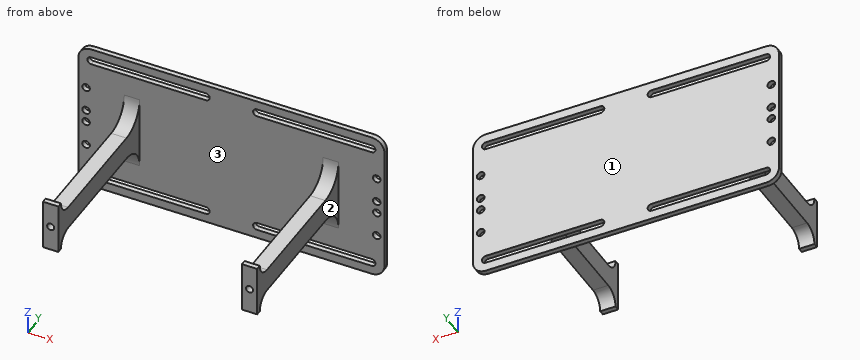
```python
from build123d import *

# Parameters (mm, degrees)
SKETCH1_W             = 6
SKETCH1_H             = 9
BOSS_EXTRUDE1_DEPTH   = 60
BOSS_EXTRUDE1_2_DEPTH = 60
SKETCH2_W             = 6
SKETCH2_H             = 20
BOSS_EXTRUDE2_DEPTH   = 2
SKETCH3_R             = 1.4
CUT_EXTRUDE1_DEPTH    = 6
FILLET1_R             = 5.5
FILLET2_R             = 5.5
SKETCH4_R             = 1.5
BOSS_EXTRUDE4_DEPTH   = 2
FILLET4_R             = 10


with BuildPart() as part:
    # Sketch1 → Boss-Extrude1 (new body)
    with BuildSketch(Plane(origin=(0, 0, 0), x_dir=(1, 0, 0), z_dir=(0, 1, 0))):
        with Locations((39, 0)):
            Rectangle(SKETCH1_W, SKETCH1_H)
    extrude(amount=BOSS_EXTRUDE1_DEPTH)



with BuildPart() as body_2:
    # Sketch1 → Boss-Extrude1 2 (new body)
    with BuildSketch(Plane(origin=(0, 0, 0), x_dir=(1, 0, 0), z_dir=(0, 1, 0))):
        with Locations((-39, 0)):
            Rectangle(SKETCH1_W, SKETCH1_H)
    extrude(amount=BOSS_EXTRUDE1_2_DEPTH)


with BuildPart() as part_1:
    add(part.part)

    add(body_2.part)  # Boss-Extrude2 merges body 2
    # Sketch2 → Boss-Extrude2 (add)
    with BuildSketch(Plane.XZ):
        with Locations((-39, 0)):
            Rectangle(SKETCH2_W, SKETCH2_H)
        with Locations((39, 0)):
            Rectangle(SKETCH2_W, SKETCH2_H)
    extrude(amount=BOSS_EXTRUDE2_DEPTH)

    # Sketch3 → Cut-Extrude1 (cut)
    with BuildSketch(Plane.XZ.offset(2)):
        with Locations(Location((39, 0, 0), (0, 0, 270))):
            Circle(SKETCH3_R)
        with Locations(Location((-39, 0, 0), (0, 0, 270))):
            Circle(SKETCH3_R)
    extrude(amount=-CUT_EXTRUDE1_DEPTH, mode=Mode.SUBTRACT)

    # Fillet1
    fillet1_edges = [part_1.edges().sort_by_distance(p)[0] for p in [
        (-39, 0, -4.5),
        (-39, 0, 4.5),
    ]]
    fillet(fillet1_edges, radius=FILLET1_R - 0.0001)  # a hair under: the kernel refuses the full size

    # Fillet2
    fillet2_edges = [part_1.edges().sort_by_distance(p)[0] for p in [
        (39, 0, -4.5),
        (39, 0, 4.5),
    ]]
    fillet(fillet2_edges, radius=FILLET2_R - 0.0001)  # a hair under: the kernel refuses the full size

    # Sketch4 → Boss-Extrude4 (add)
    with BuildSketch(Plane(origin=(0, 60, 0), x_dir=(1, 0, 0), z_dir=(0, 1, 0))):
        with BuildLine():
            Line((-55, 30), (55, 30))
            ThreePointArc((55, 30), (58.535533906, 28.535533906), (60, 25))
            Line((60, 25), (60, -25))
            ThreePointArc((60, -25), (58.535533906, -28.535533906), (55, -30))
            Line((55, -30), (-55, -30))
            ThreePointArc((-55, -30), (-58.535533906, -28.535533906), (-60, -25))
            Line((-60, -25), (-60, 25))
            ThreePointArc((-60, 25), (-58.535533906, 28.535533906), (-55, 30))
        make_face()
        with Locations(Location((-57, -2.5, 0), (0, 0, 270))):
            Circle(SKETCH4_R, mode=Mode.SUBTRACT)
        with Locations(Location((-57, -12.5, 0), (0, 0, 270))):
            Circle(SKETCH4_R, mode=Mode.SUBTRACT)
        with Locations(Location((57, -12.5, 0), (0, 0, 270))):
            Circle(SKETCH4_R, mode=Mode.SUBTRACT)
        with Locations(Location((57, -2.5, 0), (0, 0, 270))):
            Circle(SKETCH4_R, mode=Mode.SUBTRACT)
        with Locations(Location((57, 2.5, 0), (0, 0, 270))):
            Circle(SKETCH4_R, mode=Mode.SUBTRACT)
        with Locations(Location((57, 12.5, 0), (0, 0, 270))):
            Circle(SKETCH4_R, mode=Mode.SUBTRACT)
        with Locations(Location((-57, 12.5, 0), (0, 0, 270))):
            Circle(SKETCH4_R, mode=Mode.SUBTRACT)
        with Locations(Location((-57, 2.5, 0), (0, 0, 270))):
            Circle(SKETCH4_R, mode=Mode.SUBTRACT)
        with BuildLine():
            Line((55, 23.5), (10, 23.5))
            ThreePointArc((10, 23.5), (8.5, 25), (10, 26.5))
            Line((10, 26.5), (55, 26.5))
            ThreePointArc((55, 26.5), (56.5, 25), (55, 23.5))
        make_face(mode=Mode.SUBTRACT)
        with BuildLine():
            Line((-55, -23.5), (-10, -23.5))
            ThreePointArc((-10, -23.5), (-8.5, -25), (-10, -26.5))
            Line((-10, -26.5), (-55, -26.5))
            ThreePointArc((-55, -26.5), (-56.5, -25), (-55, -23.5))
        make_face(mode=Mode.SUBTRACT)
        with BuildLine():
            Line((-55, 23.5), (-10, 23.5))
            ThreePointArc((-10, 23.5), (-8.5, 25), (-10, 26.5))
            Line((-10, 26.5), (-55, 26.5))
            ThreePointArc((-55, 26.5), (-56.5, 25), (-55, 23.5))
        make_face(mode=Mode.SUBTRACT)
        with BuildLine():
            Line((55, -23.5), (10, -23.5))
            ThreePointArc((10, -23.5), (8.5, -25), (10, -26.5))
            Line((10, -26.5), (55, -26.5))
            ThreePointArc((55, -26.5), (56.5, -25), (55, -23.5))
        make_face(mode=Mode.SUBTRACT)
    extrude(amount=BOSS_EXTRUDE4_DEPTH)

    # Fillet4
    fillet4_edges = [part_1.edges().sort_by_distance(p)[0] for p in [
        (39, 60, 4.5),
        (39, 60, -4.5),
        (-39, 60, -4.5),
        (-39, 60, 4.5),
    ]]
    fillet(fillet4_edges, radius=FILLET4_R)


solid = part_1.part
```
Design review of the part built by this model. Coordinates are the model's own, in mm. Face numbers are marked on the shaded views. Give positions to 0.01 mm unless a question says otherwise; leave off trailing zeros. Write each loop counter-clockwise with the first axis right and the second up, starting at its lowest first coordinate (ties: lowest second). Pieces come first, ordered by that corner, then holes.
(1) Add section A-A (x = -39). Give the number of separate pieces and of enclosed holes in the cut face, and give its area (3 significant figures).
Checked values:
separate pieces: 3
enclosed holes: 0
area: 727 mm2
(2) Clearance check with flat-ended pins moving along their axes: pin 1 Ø1.6 at (x, y) = (-40.5, -1.5) entering from -Z; pin 2 Ø8 at (x, y) = (-45.5, 43) entering from +Z; pin 3 Ø1 at (x, y) = (38, -1) entering from +Z. State where each tip first meets the part, or that it passes through.
Checked values:
pin 1: stops at z = -10
pin 2: stops at z = 4.5
pin 3: stops at z = 10
(3) Add section D-D (x = 5). Give the boundary of the cut face in (y, z), and give its area (3 significant figures).
Checked values:
outline: (60, -30) - (62, -30) - (62, 30) - (60, 30) - close
area: 120 mm2
(4) Wall thickness on line 1 along X through (y, z) = (0.25, 0); line 2 along X through (y, z) = (60.5, -12.5); line 3 along X through (y, z) = (19.5, -0.5): over which ranges is each line inside the solid? List them lowest first.
Checked values:
line 1: x = -42 to -40.4, -37.6 to -36, 36 to 37.6, 40.4 to 42
line 2: x = -60 to -58.5, -55.5 to 55.5, 58.5 to 60
line 3: x = -42 to -36, 36 to 42
(5) Add section B-B (z = 12.5). Give the boundary of the cut face in (x, y).
Checked values:
outline: (-60, 60) - (-58.5, 60) - (-58.5, 62) - (-60, 62) - close; (-55.5, 60) - (-42, 60) - (-42, 59.8) - (-36, 59.8) - (-36, 60) - (36, 60) - (36, 59.8) - (42, 59.8) - (42, 60) - (55.5, 60) - (55.5, 62) - (-55.5, 62) - close; (58.5, 60) - (60, 60) - (60, 62) - (58.5, 62) - close
(6) Add section C-C (x = -12.5). Give the boundary of the cut face in (y, z).
Checked values:
outline: (60, -30) - (62, -30) - (62, -26.5) - (60, -26.5) - close; (60, -23.5) - (62, -23.5) - (62, 23.5) - (60, 23.5) - close; (60, 26.5) - (62, 26.5) - (62, 30) - (60, 30) - close
(7) Mouldability with a two-part tool opening along X and no side actions: class the marked faces 1, 2 and 3 as +X half, -X half, draft (parallel to the pull), parting line (faces both ways), or undercut.
Checked values:
face 1: draft
face 2: +X half
face 3: undercut
